CAD build for the part. Positions are in the model's coordinates, mm. A direction names the side the tool comes from. Round coordinates to 2 decimals unless told otherwise and drop trailing zeros. Loops run counter-clockwise (first coordinate to the right, second up) from the corner with the lowest first, then second, coordinate; pieces in that order, holes last. Notation, with made-up numbers: M -11.5,72.25 L 14.5,72.25 A15 ccw 14.5,91.25 Z; hole C 21.5,-27.75 d7. An arc over 180 degrees is marked long. Use a Markdown table: item, result. Add a question column.
(1) Two-plate mould, pull along X, no slides. Class faces 5 (the face through (-28, 112.333, 9)), 6 (the face through (160.176, 5.851, 2.958)), 7 (the face through (-45.147, 33, 9)), 8 (the face through (-30.81, 100.34, 6.08)): released by +X, released by -X, zero draft, split by the parting line, or undercut.
(2) Wall check: L1, parallel to Y at x = -21.5, z = 2; L2, parallel to X at y = 59.5, z = 11.5; L3, parallel to Z at x = 100.5, y = 106. Give the ranges that are in metal, low to high.
(3) Band-saw the part on C-C, the plane x = 32. Write the cut outline in (y, z).
(4) Band-saw the part on A-A, the plane x = -28. Write the cut outline in (y, z).
(5) Band-saw the part on B-B, the plane y = -30. Write the cut outline in (x, z), and give its area (3 significant figures).
(6) Which spindle directions (+Z, -Z, +X, -X, +Y, -Y) get a long thin tool onto all of the face, cutting with end or side? Do faces 1 (the face through (141.983, -31, 9)), 2 (the face through (-55.686, 42, 3)), 3 (the face through (47, -43.866, 9)), 4 (the face through (-10.477, 46, 9)). Say none if no direction does.
(7) Flat gauge pins, fed straight in: P1, Ø20, axis at x = -29.41, y = -22.36, coming from the +Z side; P2, Ø3, axis at y = 68, z = 9, coming from the -X side; P3, Ø3, axis at y = 97.5, z = 5.5, coming from the +X side; P4, Ø6.5, axis at x = 60, z = 10, coming from the +Y side. Where does each tip first touch, or does it go through?
(8) Band-saw the part on D-D, the plane z = 4. Write the cut outline in (x, y).
from build123d import *

# Parameters (mm, degrees)
SALIENTE_EXTRUIR1_DEPTH = 6
CROQUIS2_W              = 34.669355488
CROQUIS2_H              = 156.198494079
SALIENTE_EXTRUIR2_DEPTH = 6
CROQUIS4_W              = 152.460808534
CROQUIS4_H              = 25.435907393
SALIENTE_EXTRUIR3_DEPTH = 6
CROQUIS5_R              = 11.076486621
CROQUIS5_R_2            = 10.775241997
CORTAR_EXTRUIR1_DEPTH   = 12


with BuildPart() as part:
    # Croquis1 → Saliente-Extruir1 (new body)
    with BuildSketch(Plane.XY):
        Polygon((182.356839795, 53.079696336), (196.865539042, 88.764755078), (208.451032663, 111.909466833), (208.451032663, 130.571133231), (182.356839795, 130.571133231), (-55.686414529, 130.571133231), (-55.686414529, -49.428866769), (144.313585471, -49.428866769), (152.562750691, -5.750074162), (168.005565446, 17.781834037), align=None)
    extrude(amount=SALIENTE_EXTRUIR1_DEPTH)

    # Croquis2 → Saliente-Extruir2 (add)
    with BuildSketch(Plane.XY.offset(6)):
        with Locations((-27.81215178, 34.233724164)):
            Rectangle(CROQUIS2_W, CROQUIS2_H)
    extrude(amount=SALIENTE_EXTRUIR2_DEPTH)

    # Croquis4 → Saliente-Extruir3 (add)
    with BuildSketch(Plane.XY.offset(6)):
        with Locations((65.752930231, -31.14756918)):
            Rectangle(CROQUIS4_W, CROQUIS4_H)
    extrude(amount=SALIENTE_EXTRUIR3_DEPTH)

    # Croquis5 → Cortar-Extruir1 (cut)
    with BuildSketch(Plane.XY.offset(12)):
        with Locations((-29.411710595, -22.364568106)):
            Circle(CROQUIS5_R)
        with Locations((-29.411710595, 89.657796537)):
            Circle(CROQUIS5_R_2)
    extrude(amount=-CORTAR_EXTRUIR1_DEPTH, mode=Mode.SUBTRACT)


solid = part.part
Return value:
| question | item | result |
|---|---|---|
| 1 | face 5 | zero draft |
| 1 | face 6 | released by +X |
| 1 | face 7 | released by -X |
| 1 | face 8 | undercut |
| 2 | L1 | -49.43 to -30.12, -14.61 to 82.34, 96.97 to 130.57 |
| 2 | L2 | -45.15 to -10.48 |
| 2 | L3 | 0 to 6 |
| 3 | outline | M -49.43,0 L 130.57,0 L 130.57,6 L -18.43,6 L -18.43,12 L -43.87,12 L -43.87,6 L -49.43,6 Z |
| 4 | outline | M -49.43,0 L -33.35,0 L -33.35,12 L -43.87,12 L -43.87,6 L -49.43,6 Z; M -11.38,0 L 78.98,0 L 78.98,12 L -11.38,12 Z; M 100.34,0 L 130.57,0 L 130.57,6 L 112.33,6 L 112.33,12 L 100.34,12 Z |
| 5 | outline | M -55.69,0 L -37.44,0 L -37.44,12 L -45.15,12 L -45.15,6 L -55.69,6 Z; M -21.39,0 L 147.98,0 L 147.98,6 L 141.98,6 L 141.98,12 L -21.39,12 Z |
| 5 | area | 2,150 mm^2 |
| 6 | face 1 | +Z, +X, +Y, -Y |
| 6 | face 2 | +Z, -Z, -X, +Y, -Y |
| 6 | face 3 | +Z, +X, -X, -Y |
| 6 | face 4 | +Z, +X, +Y |
| 7 | P1 | through |
| 7 | P2 | x = -45.15 |
| 7 | P3 | x = 201.99 |
| 7 | P4 | y = -18.43 |
| 8 | outline | M -55.69,-49.43 L 144.31,-49.43 L 152.56,-5.75 L 168.01,17.78 L 196.87,88.76 L 208.45,111.91 L 208.45,130.57 L -55.69,130.57 Z; hole C -29.41,-22.36 d22.15; hole C -29.41,89.66 d21.55 |
